Geometry: final body of the model. Coordinates: model frame, mm. A direction names the side the tool comes from. Give positions to 0.01 mm unless a question says otherwise; leave off trailing zeros. Loops run counter-clockwise (first coordinate to the right, second up) from the corner with the lowest first, then second, coordinate; pieces in that order, holes last.
from build123d import *

# Parameters (mm, degrees)
SKETCH1_W           = 40
SKETCH1_H           = 40
BOSS_EXTRUDE1_DEPTH = 10
FILLET1_R           = 1
SKETCH2_R           = 18
SKETCH2_R_2         = 7
CUT_EXTRUDE2_DEPTH  = 10
SKETCH3_R           = 1.6
CUT_EXTRUDE3_DEPTH  = 11
BOSS_EXTRUDE2_DEPTH = 1
FILLET2_R           = 1
FILLET3_R           = 1
FILLET4_R           = 0.3


with BuildPart() as part:
    # Sketch1 → Boss-Extrude1 (new body)
    with BuildSketch(Plane(origin=(0, 0, 0), x_dir=(1, 0, 0), z_dir=(0, 1, 0))):
        with Locations((-20, 20)):
            Rectangle(SKETCH1_W, SKETCH1_H)
    extrude(amount=BOSS_EXTRUDE1_DEPTH)

    # Fillet1
    fillet1_edges = [part.edges().sort_by_distance(p)[0] for p in [
        (0, 5, 0),
        (-40, 5, 0),
        (-40, 5, -40),
        (0, 5, -40),
    ]]
    fillet(fillet1_edges, radius=FILLET1_R)

    # Sketch2 → Cut-Extrude2 (cut)
    with BuildSketch(Plane(origin=(0, 10, 0), x_dir=(1, 0, 0), z_dir=(0, 1, 0))):
        with Locations((-20, 20)):
            Circle(SKETCH2_R)
        with Locations((-20, 20)):
            Circle(SKETCH2_R_2, mode=Mode.SUBTRACT)
    extrude(amount=-CUT_EXTRUDE2_DEPTH, mode=Mode.SUBTRACT)

    # Sketch3 → Cut-Extrude3 (cut, through all)
    with BuildSketch(Plane(origin=(0, 10, 0), x_dir=(1, 0, 0), z_dir=(0, 1, 0))):
        with Locations((-36, 36)):
            Circle(SKETCH3_R)
        with Locations((-4, 36)):
            Circle(SKETCH3_R)
        with Locations((-4, 4)):
            Circle(SKETCH3_R)
        with Locations((-36, 4)):
            Circle(SKETCH3_R)
    extrude(amount=-CUT_EXTRUDE3_DEPTH, mode=Mode.SUBTRACT)

    # Sketch7 → Boss-Extrude2 (add)
    with BuildSketch(Plane(origin=(0, 10, 0), x_dir=(1, 0, 0), z_dir=(0, 1, 0))):
        with BuildLine():
            Line((-21, 21), (-37.972200756, 21))
            ThreePointArc((-37.972200756, 21), (-38, 20), (-37.972200756, 19))
            Line((-37.972200756, 19), (-21, 19))
            Line((-21, 19), (-21, 21))
        make_face()
        with BuildLine():
            Line((-21, 37.972200756), (-21, 21))
            Line((-21, 21), (-19, 21))
            Line((-19, 21), (-19, 37.972200756))
            ThreePointArc((-19, 37.972200756), (-20, 38), (-21, 37.972200756))
        make_face()
        with BuildLine():
            Line((-2.027799244, 21), (-19, 21))
            Line((-19, 21), (-19, 19))
            Line((-19, 19), (-2.027799244, 19))
            ThreePointArc((-2.027799244, 19), (-2.006951153, 19.499806838), (-2, 20))
            ThreePointArc((-2, 20), (-2.006951153, 20.500193162), (-2.027799244, 21))
        make_face()
        with BuildLine():
            Line((-19, 19), (-21, 19))
            Line((-21, 19), (-21, 2.027799244))
            ThreePointArc((-21, 2.027799244), (-20, 2), (-19, 2.027799244))
            Line((-19, 2.027799244), (-19, 19))
        make_face()
    extrude(amount=-BOSS_EXTRUDE2_DEPTH)

    # Fillet2
    fillet2_edges = [part.edges().sort_by_distance(p)[0] for p in [
        (-27, 0, -20),
    ]]
    fillet(fillet2_edges, radius=FILLET2_R)

    # Fillet3
    fillet3_edges = [part.edges().sort_by_distance(p)[0] for p in [
        (-38, 0, -20),
    ]]
    fillet(fillet3_edges, radius=FILLET3_R)

    # Fillet4
    fillet4_edges = [part.edges().sort_by_distance(p)[0] for p in [
        (0, 0, -20),
        (-20, 0, -40),
        (-40, 0, -20),
        (-20, 0, 0),
        (-0.292893219, 0, -39.707106781),
        (-0.292893219, 0, -0.292893219),
        (-39.707106781, 0, -0.292893219),
        (-39.707106781, 0, -39.707106781),
    ]]
    fillet(fillet4_edges, radius=FILLET4_R)


solid = part.part
Item 1: Set-up query: faces 4 (the face through (-20, 9, -8)), 5 (the face through (-32.5, 9.5, -19)), 6 (the face through (-39.715, 5.218, -39.699)). Return all of +Z, -Z, +X, -X, +Y, -Y with unobstructed straight access to the full face (end or side cutting, diameter ignored); none if empty.
Values follow:
face 4: -Y
face 5: +Y, -Y
face 6: -Z, -X, +Y, -Y
Item 2: Pin query (flat end, axial travel): pin 1 (3 mm diameter, centred on x = -36, z = -4, fed in from -Y); pin 2 (1 mm diameter, centred on x = -20.5, z = -33.5, fed in from -Y). Return the tip coordinate at first contact, or that it passes through.
Values follow:
pin 1: passes through
pin 2: stops at y = 9
Item 3: Section query C-C on x = -20. Return loops of the section in (y, z), plus the area to 3 significant figures.
Values follow:
outline: (0, -39.7) arc R0.3 ccw to (0.3, -40) - (10, -40) - (10, 0) - (0.3, 0) arc R0.3 ccw to (0, -0.3) - (0, -1) arc R1 ccw to (1, -2) - (9, -2) - (9, -13) - (1, -13) arc R1 ccw to (0, -14) - (0, -26) arc R1 ccw to (1, -27) - (9, -27) - (9, -38) - (1, -38) arc R1 ccw to (0, -39) - close
area: 201 mm2
Item 4: Section query B-B on z = -20. Return loops of the section in (x, y).
Values follow:
outline: (-40, 0.3) arc R0.3 ccw to (-39.7, 0) - (-39, 0) arc R1 ccw to (-38, 1) - (-38, 9) - (-27, 9) - (-27, 1) arc R1 ccw to (-26, 0) - (-14, 0) arc R1 ccw to (-13, 1) - (-13, 9) - (-2, 9) - (-2, 1) arc R1 ccw to (-1, 0) - (-0.3, 0) arc R0.3 ccw to (0, 0.3) - (0, 10) - (-40, 10) - close
Item 5: Section query D-D on x = -7.5. Give the number of separate pieces and of enclosed holes in the cut face, plus the area to 3 significant figures.
Values follow:
separate pieces: 3
enclosed holes: 0
area: 142 mm2
Item 6: Ray query, probe 1 along X at (y, z) = (4.5, -20); probe 2 along Z at (x, y) = (-36.5, 6.75). Return the intervals inside material, ascending.
Values follow:
probe 1: x = -40 to -38, -27 to -13, -2 to 0
probe 2: z = -40 to -37.52, -34.48 to -27.19, -12.81 to -5.52, -2.48 to 0
Item 7: Section query A-A on y = 4.75. Return loops of the section in (x, z), plus the area to 3 significant figures.
Values follow:
outline: (-40, -39) arc R1 ccw to (-39, -40) - (-1, -40) arc R1 ccw to (0, -39) - (0, -1) arc R1 ccw to (-1, 0) - (-39, 0) arc R1 ccw to (-40, -1) - close; circle Ø14 at (-20, -20); hole circle Ø36 at (-20, -20); hole circle Ø3.2 at (-36, -36); hole circle Ø3.2 at (-36, -4); hole circle Ø3.2 at (-4, -36); hole circle Ø3.2 at (-4, -4)
area: 703 mm2
Item 8: Draft query along Z for faces 1 (the face through (-3.26, 5.07, -34.58)), 2 (the face through (-39.715, 5.218, -0.301)), 3 (the face through (-20, 5, -40)). Return one class per face: +Z half, -Z half, draft (parallel to the pull), parting line (faces both ways), or undercut.
Values follow:
face 1: undercut
face 2: +Z half
face 3: -Z half
